Can you work these out from the model? Positions are in its coordinate system, mm. A direction names the side the tool comes from. Round coordinates to 2 decimals unless told otherwise and drop trailing zeros. Order: outer loops, then holes, each group sorted by start corner. A loop starts at its lowest first (then second) coordinate and runs counter-clockwise, first axis right, second up. Notation, with made-up numbers: (46, 70) -> (58, 70) arc R17 ccw to (58, 100) -> close; hole circle Ø9 at (-15.75, 9). An arc over 180 degrees is marked (long way). Use a Markdown table: item, result. Add a question column.
Q1. If we section it at A-A on y = 39: List the corners of the cut face in (x, z) for me.
Q2. I need wall thicknesses on line 1 along Y through (x, z) = (5, 1.8); line 2 along Z through (x, y) = (2.25, 43.5); line 3 along Y through (x, z) = (11, -12). Which ranges of each line are inside material? Lowest first, please. Write a range as [from, to].
Q3. If we section it at C-C on x = 10.5: List the corners of the cut face in (y, z) for me, plus the area to 3 significant figures.
Q4. If we section it at B-B on z = 12.5: List the corners of the cut face in (x, y) for me, plus the area to 4 significant figures.
Q5. We'd pull the mould along Z, two halves only. Please class faces 1 (the face through (-4.595, 54.493, 16.198)), 2 (the face through (3.59, 53.43, 5.6)), 3 (the face through (-7.5, 64, -15)): +Z half, -Z half, draft (parallel to the pull), parting line (faces both ways), or undercut.
Q6. I'm going to push flat-ended pins straight in: pin 1 Ø10.5 at (x, y) = (9.5, 46) entering from +Z; pin 2 Ø4.5 at (x, y) = (5, 47) entering from -Z; pin 3 Ø6.5 at (x, y) = (0, 37.5) entering from -Z; pin 4 Ø9.5 at (x, z) = (-4.5, 10.5) entering from -Y. Where does each tip first touch, or does it pass through?
Q7. If we section it at D-D on y = 47: List the corners of the cut face in (x, z) for me.
Q8. For faces 4 (the face through (6, 54, 12)), 5 (the face through (-4.655, 54.493, 8.837)), 6 (the face through (-3.841, 64.507, -14.267)), 7 (the face through (-3.7, 63, 10.9)), 8 (the face through (4, 41, -10)), which set-ups out of +Z, -Z, +X, -X, +Y, -Y let a thin tool reach every point of the face, with its end or its side?
```python
from build123d import *

# Parameters (mm, degrees)
SKETCH2_W            = 10
SKETCH2_H            = 21
SKETCH2_R            = 2.5
BOSS_EXTRUDE1_DEPTH  = 5
BOSS_EXTRUDE3_START  = 5
SKETCH3_W            = 10
SKETCH3_H            = 21
SKETCH3_R            = 2.5
BOSS_EXTRUDE3_DEPTH  = 5
SKETCH4_W            = 10
SKETCH4_H            = 5
BOSS_EXTRUDE4_DEPTH  = 2
SKETCH5_W            = 10
SKETCH5_H            = 5
BOSS_EXTRUDE5_DEPTH  = 2
BOSS_EXTRUDE6_DEPTH  = 3
FILLET1_R            = 1
FILLET2_R            = 2
BOSS_EXTRUDE7_DEPTH  = 5
SKETCH9_W            = 2
SKETCH9_H            = 40
BOSS_EXTRUDE8_DEPTH  = 5
SKETCH10_W           = 15
SKETCH10_H           = 40
BOSS_EXTRUDE9_DEPTH  = 3
CUT_EXTRUDE1_DEPTH   = 3
SKETCH13_W           = 14.256248666
SKETCH13_H           = 3
BOSS_EXTRUDE10_DEPTH = 7.5
SKETCH14_R           = 2
CUT_EXTRUDE2_DEPTH   = 44.44249072
SKETCH15_R           = 3.5
CUT_EXTRUDE3_DEPTH   = 1
CUT_EXTRUDE4_DEPTH   = 1
CUT_EXTRUDE5_DEPTH   = 1
FILLET3_R            = 5
FILLET4_R            = 2
FILLET5_R            = 2


with BuildPart() as part:
    # Sketch2 → Boss-Extrude1 (new body)
    with BuildSketch(Plane.XY):
        with Locations((5, 41.5)):
            Rectangle(SKETCH2_W, SKETCH2_H)
        with Locations((5, 47)):
            Circle(SKETCH2_R, mode=Mode.SUBTRACT)
        with Locations((5, 37)):
            Circle(SKETCH2_R, mode=Mode.SUBTRACT)
    extrude(amount=BOSS_EXTRUDE1_DEPTH)

    # Sketch4 → Boss-Extrude4 (add)
    with BuildSketch(Plane(origin=(0, 52, 0), x_dir=(1, 0, 0), z_dir=(0, 1, 0))):
        with Locations((5, -2.5)):
            Rectangle(SKETCH4_W, SKETCH4_H)
    extrude(amount=BOSS_EXTRUDE4_DEPTH)



with BuildPart() as body_2:
    # Sketch3 → Boss-Extrude3 (new body)
    with BuildSketch(Plane(origin=(0, 0, 0), x_dir=(-1, 0, 0), z_dir=(0, 0, -1)).offset(BOSS_EXTRUDE3_START)):
        with Locations((-5, 41.5)):
            Rectangle(SKETCH3_W, SKETCH3_H)
        with Locations(Location((-5, 37, 0), (0, 0, 180))):
            Circle(SKETCH3_R, mode=Mode.SUBTRACT)
        with Locations(Location((-5, 47, 0), (0, 0, 180))):
            Circle(SKETCH3_R, mode=Mode.SUBTRACT)
    extrude(amount=BOSS_EXTRUDE3_DEPTH)

    # Sketch5 → Boss-Extrude5 (add)
    with BuildSketch(Plane(origin=(0, 52, 0), x_dir=(1, 0, 0), z_dir=(0, 1, 0))):
        with Locations((5, 7.5)):
            Rectangle(SKETCH5_W, SKETCH5_H)
    extrude(amount=BOSS_EXTRUDE5_DEPTH)


with BuildPart() as part_1:
    add(part.part)

    add(body_2.part)  # Boss-Extrude6 merges body 2
    # Sketch6 → Boss-Extrude6 (add)
    with BuildSketch(Plane(origin=(0, 54, 0), x_dir=(1, 0, 0), z_dir=(0, 1, 0))):
        Polygon((10, -5), (10, -17.5), (0, -17.5), (0, -5), (0, 10), (0, 22.5), (10, 22.5), (10, 10), align=None)
    extrude(amount=BOSS_EXTRUDE6_DEPTH)

    # Fillet1
    fillet1_edges = [part_1.edges().sort_by_distance(p)[0] for p in [
        (5, 54, 0),
        (5, 54, -5),
    ]]
    fillet(fillet1_edges, radius=FILLET1_R)

    # Fillet2
    fillet2_edges = [part_1.edges().sort_by_distance(p)[0] for p in [
        (5, 54, 5),
        (5, 54, -10),
    ]]
    fillet(fillet2_edges, radius=FILLET2_R)

    # Sketch8 → Boss-Extrude7 (add)
    with BuildSketch(Plane(origin=(10, 0, 0), x_dir=(0, 0, -1), z_dir=(1, 0, 0))):
        with BuildLine():
            Line((0, 31), (0, 53))
            ThreePointArc((0, 53), (0.292893219, 53.707106781), (1, 54))
            Line((1, 54), (4, 54))
            ThreePointArc((4, 54), (4.707106781, 53.707106781), (5, 53))
            Line((5, 53), (5, 31))
            Line((5, 31), (10, 31))
            Line((10, 31), (10, 52))
            ThreePointArc((10, 52), (10.585786438, 53.414213562), (12, 54))
            Line((12, 54), (22.5, 54))
            Line((22.5, 54), (22.5, 57))
            Line((22.5, 57), (-17.5, 57))
            Line((-17.5, 57), (-17.5, 54))
            Line((-17.5, 54), (-7, 54))
            ThreePointArc((-7, 54), (-5.585786438, 53.414213562), (-5, 52))
            Line((-5, 52), (-5, 31))
            Line((-5, 31), (0, 31))
        make_face()
    extrude(amount=BOSS_EXTRUDE7_DEPTH)

    # Sketch9 → Boss-Extrude8 (add)
    with BuildSketch(Plane(origin=(0, 57, 0), x_dir=(1, 0, 0), z_dir=(0, 1, 0))):
        with Locations((14, 2.5)):
            Rectangle(SKETCH9_W, SKETCH9_H)
    extrude(amount=BOSS_EXTRUDE8_DEPTH)

    # Sketch10 → Boss-Extrude9 (add)
    with BuildSketch(Plane(origin=(0, 62, 0), x_dir=(1, 0, 0), z_dir=(0, 1, 0))):
        with Locations((7.5, 2.5)):
            Rectangle(SKETCH10_W, SKETCH10_H)
    extrude(amount=BOSS_EXTRUDE9_DEPTH)

    # Sketch12 → Cut-Extrude1 (cut)
    with BuildSketch(Plane(origin=(0, 65, 0), x_dir=(1, 0, 0), z_dir=(0, 1, 0))):
        Polygon((13, 8.243751334), (2, 8.243751334), (0, 8.243751334), (0, -3.243751334), (2, -3.243751334), (13, -3.243751334), align=None)
    extrude(amount=-CUT_EXTRUDE1_DEPTH, mode=Mode.SUBTRACT)

    # Sketch13 → Boss-Extrude10 (add)
    with BuildSketch(Plane.ZY):
        with Locations((10.371875667, 63.5)):
            Rectangle(SKETCH13_W, SKETCH13_H)
        with BuildLine():
            Line((-4, 54), (-1, 54))
            ThreePointArc((-1, 54), (-0.292893219, 53.707106781), (0, 53))
            Line((0, 53), (0, 31))
            Line((0, 31), (5, 31))
            Line((5, 31), (5, 52))
            ThreePointArc((5, 52), (5.585786438, 53.414213562), (7, 54))
            Line((7, 54), (17.5, 54))
            Line((17.5, 54), (17.5, 57))
            Line((17.5, 57), (-22.5, 57))
            Line((-22.5, 57), (-22.5, 54))
            Line((-22.5, 54), (-12, 54))
            ThreePointArc((-12, 54), (-10.585786438, 53.414213562), (-10, 52))
            Line((-10, 52), (-10, 31))
            Line((-10, 31), (-5, 31))
            Line((-5, 31), (-5, 53))
            ThreePointArc((-5, 53), (-4.707106781, 53.707106781), (-4, 54))
        make_face()
        with Locations((-15.371875667, 63.5)):
            Rectangle(SKETCH13_W, SKETCH13_H)
    extrude(amount=BOSS_EXTRUDE10_DEPTH)

    # Sketch14 → Cut-Extrude2 (cut, through all)
    with BuildSketch(Plane(origin=(0, 65, 0), x_dir=(1, 0, 0), z_dir=(0, 1, 0))):
        with Locations(Location((-2.5, -12.5, 0), (0, 0, 270))):
            Circle(SKETCH14_R)
        with Locations(Location((-2.5, 17.5, 0), (0, 0, 270))):
            Circle(SKETCH14_R)
    extrude(amount=-CUT_EXTRUDE2_DEPTH, mode=Mode.SUBTRACT)

    # Sketch15 → Cut-Extrude3 (cut)
    with BuildSketch(Plane(origin=(0, 65, 0), x_dir=(1, 0, 0), z_dir=(0, 1, 0))):
        with Locations(Location((-2.5, 17.5, 0), (0, 0, 270))):
            Circle(SKETCH15_R)
        with Locations(Location((-2.5, -12.5, 0), (0, 0, 270))):
            Circle(SKETCH15_R)
    extrude(amount=-CUT_EXTRUDE3_DEPTH, mode=Mode.SUBTRACT)

    # Sketch16 → Cut-Extrude4 (cut)
    with BuildSketch(Plane.XZ.offset(-54)):
        Polygon((-6.75, 14.953738644), (-6.75, 10.046261356), (-2.5, 7.592522712), (1.75, 10.046261356), (1.75, 14.953738644), (-2.5, 17.407477288), align=None)
    extrude(amount=-CUT_EXTRUDE4_DEPTH, mode=Mode.SUBTRACT)

    # Sketch17 → Cut-Extrude5 (cut)
    with BuildSketch(Plane(origin=(0, 54, 0), x_dir=(-1, 0, 0), z_dir=(0, -1, 0))):
        Polygon((6.75, 15.046261356), (6.75, 19.953738644), (2.5, 22.407477288), (-1.75, 19.953738644), (-1.75, 15.046261356), (2.5, 12.592522712), align=None)
    extrude(amount=-CUT_EXTRUDE5_DEPTH, mode=Mode.SUBTRACT)

    # Fillet3
    fillet3_edges = [part_1.edges().sort_by_distance(p)[0] for p in [
        (-7.5, 31, 2.5),
        (-7.5, 31, -7.5),
    ]]
    fillet(fillet3_edges, radius=FILLET3_R)

    # Fillet4
    fillet4_edges = [part_1.edges().sort_by_distance(p)[0] for p in [
        (-7.5, 55.5, 17.5),
        (-7.5, 55.5, -22.5),
        (-7.5, 63.5, 17.5),
        (-7.5, 63.5, 3.243751334),
        (-7.5, 63.5, -22.5),
        (-7.5, 63.5, -8.243751334),
    ]]
    fillet(fillet4_edges, radius=FILLET4_R)

    # Fillet5
    fillet5_edges = [part_1.edges().sort_by_distance(p)[0] for p in [
        (13, 63.5, -8.243751334),
        (13, 63.5, 3.243751334),
    ]]
    fillet(fillet5_edges, radius=FILLET5_R)


solid = part_1.part
```
Answer below:
| question | item | result |
|---|---|---|
| 1 | outline | (-7.5, -10) -> (3.5, -10) -> (3.5, -5) -> (-7.5, -5) -> close; (-7.5, 0) -> (3.5, 0) -> (3.5, 5) -> (-7.5, 5) -> close; (6.5, -10) -> (15, -10) -> (15, -5) -> (6.5, -5) -> close; (6.5, 0) -> (15, 0) -> (15, 5) -> (6.5, 5) -> close |
| 2 | line 1 | [31, 34.5], [39.5, 44.5], [49.5, 57] |
| 2 | line 2 | [-10, -5], [0, 5] |
| 2 | line 3 | [54, 57], [62, 65] |
| 3 | outline | (31, -10) -> (52, -10) arc R2 cw to (54, -12) -> (54, -22.5) -> (57, -22.5) -> (57, 17.5) -> (54, 17.5) -> (54, 7) arc R2 cw to (52, 5) -> (31, 5) -> (31, 0) -> (53, 0) arc R1 cw to (54, -1) -> (54, -4) arc R1 cw to (53, -5) -> (31, -5) -> close; (62, -22.5) -> (65, -22.5) -> (65, -8.24) -> (62, -8.24) -> close; (62, 3.24) -> (65, 3.24) -> (65, 17.5) -> (62, 17.5) -> close |
| 3 | area | 438 mm² |
| 4 | outline | (-7.5, 54) -> (-6.75, 54) -> (-6.75, 55) -> (-4.5, 55) -> (-4.5, 57) -> (-7.5, 57) -> close; (-7.5, 62) -> (-4.5, 62) -> (-4.5, 64) -> (-6, 64) -> (-6, 65) -> (-7.5, 65) -> close; (-0.5, 55) -> (1.75, 55) -> (1.75, 54) -> (15, 54) -> (15, 65) -> (1, 65) -> (1, 64) -> (-0.5, 64) -> (-0.5, 62) -> (13, 62) -> (13, 57) -> (-0.5, 57) -> close |
| 4 | area | 113.5 mm² |
| 5 | face 1 | undercut |
| 5 | face 2 | +Z half |
| 5 | face 3 | draft |
| 6 | pin 1 | z = 5 |
| 6 | pin 2 | through |
| 6 | pin 3 | z = -10 |
| 6 | pin 4 | y = 53.56 |
| 7 | outline | (-7.5, -10) -> (2.5, -10) -> (2.5, -5) -> (-7.5, -5) -> close; (-7.5, 0) -> (2.5, 0) -> (2.5, 5) -> (-7.5, 5) -> close; (7.5, -10) -> (15, -10) -> (15, -5) -> (7.5, -5) -> close; (7.5, 0) -> (15, 0) -> (15, 5) -> (7.5, 5) -> close |
| 8 | face 4 | +Z, +X, -X, -Y |
| 8 | face 5 | -Y |
| 8 | face 6 | +Y |
| 8 | face 7 | +Y, -Y |
| 8 | face 8 | -Z, +X, -X, -Y |
